Work out the finished part from the listing and answer in its coordinate system (mm). Round coordinates to 2 decimals unless told otherwise and drop trailing zeros. Order: outer loops, then holes, each group sorted by start corner. A loop starts at its lowest first (then second) coordinate and runs counter-clockwise, first axis right, second up. Notation, with made-up numbers: (17, 15) - (38, 15) arc R25 cw to (38, 54) - close; hole circle Ø10 at (25, -37). An arc over 180 degrees is marked (long way). Put each result on its own line as item: value.
```python
from build123d import *

# Parameters (mm, degrees)
F0_W     = 232
F0_H     = 85
F2_DEPTH = 3
F3_W     = 212
F3_H     = 65
F4_DEPTH = 3
F5_R     = 12
F6_R     = 1.85
F7_DEPTH = 3


# Not quite as in the source:
# - a feature names something its author has since deleted; it is built from what else it names


with BuildPart() as f2:
    # F0 (on Top) → F2 (new body)
    with BuildSketch(Plane.XY):
        Rectangle(F0_W, F0_H)
    extrude(amount=F2_DEPTH)

    # F3 (on face) → F4 (cut)
    with BuildSketch(Plane.XY.offset(3)):
        Rectangle(F3_W, F3_H)
    extrude(amount=-F4_DEPTH, mode=Mode.SUBTRACT)

    # F5
    f5_edges = [f2.edges().sort_by_distance(p)[0] for p in [
        (-106, -32.5, 1.5),
        (106, -32.5, 1.5),
    ]]
    fillet(f5_edges, radius=F5_R)

    # F6 (on face) → F7 (cut)
    with BuildSketch(Plane.XY.offset(3)):
        with Locations((-108.5, -35)):
            Circle(F6_R)
        with Locations((108.5, -35)):
            Circle(F6_R)
    extrude(amount=-F7_DEPTH, mode=Mode.SUBTRACT)


solid = f2.part
```
1) A cutting plane is placed at B-B on y = 30.5. Write down the section's boundary in (x, z).
Findings below:
outline: (-116, 0) - (-106, 0) - (-106, 3) - (-116, 3) - close; (106, 0) - (116, 0) - (116, 3) - (106, 3) - close
2) A cutting plane is placed at A-A on z = 2.45. Write down the section's boundary in (x, y).
Findings below:
outline: (-116, -42.5) - (116, -42.5) - (116, 42.5) - (-116, 42.5) - close; hole circle Ø3.7 at (-108.5, -35); hole (-106, -20.5) arc R12 ccw to (-94, -32.5) - (94, -32.5) arc R12 ccw to (106, -20.5) - (106, 32.5) - (-106, 32.5) - close; hole circle Ø3.7 at (108.5, -35)
3) Straight lines are drawn through the part: L1, parallel to Y at x = 16, z = 0.6; L2, parallel to X at y = -2, z = 1.55; L3, parallel to Y at x = 108.5, z = 2.45. For each, find the intervals that lie inside material, in ascending order. Write a range as from..to.
Findings below:
L1: y = -42.5..-32.5, 32.5..42.5
L2: x = -116..-106, 106..116
L3: y = -42.5..-36.85, -33.15..42.5
4) For a pull along X with two mould halves and no side action, classify faces 1 (the cylindrical face through (-102.39, -29.08, 1.48)), 2 (the flat face through (-1, 35, 3)), 3 (the cylindrical face through (102.39, -29.08, 1.48)) as pulls with the +X half, pulls with the -X half, needs draft (parallel to the pull), parting line crosses it, or undercut.
Findings below:
face 1: undercut
face 2: needs draft
face 3: undercut
5) A cutting plane is placed at C-C on x = -91.5. Write down the section's boundary in (y, z), then the cut area to 3 significant figures.
Findings below:
outline: (-42.5, 0) - (-32.5, 0) - (-32.5, 3) - (-42.5, 3) - close; (32.5, 0) - (42.5, 0) - (42.5, 3) - (32.5, 3) - close
area: 60.0 mm2
6) Given pin 1 Ø3.5 at (x, y) = (108.5, -35) entering from -Z, flat-ended and moving along its own axis, determine where the tip first touches the part or whether it passes through.
Findings below:
pin 1: passes through
